CAD build for the part. Positions are in the model's coordinates, mm. Face numbers are marked on the shaded views. Give positions to 0.01 mm unless a question says otherwise; leave off trailing zeros. Loops run counter-clockwise (first coordinate to the right, second up) from the corner with the lowest first, then second, coordinate; pieces in that order, holes last.
Item 1: Mould opens along Z. For the marked faces 1, 2 and 3 say: released by +Z, released by -Z, zero draft, split by the parting line, or undercut.
Item 2: Saw through at C-C on x = -15.5. Give the cut face in (y, z).
Item 3: Saw through at B-B on z = 3. Give the cut face in (x, y), plus the area to 3 significant figures.
Item 4: Drop a flat-ended pin along its axis: P1, Ø4, axis at x = -15.5, z = -24.9, coming from the -Y side. Give the stop position or say it passes through.
Item 5: Probe probe 1 along X at (y, z) = (3.25, -14); probe 2 along Z at (x, y) = (25, 2.3); probe 3 along Z at (x, y) = (14.5, 4.5). List the from-to ranges inside material, lowest first.
Item 6: Saw through at A-A on x = -6.5. Give the cut face in (y, z).
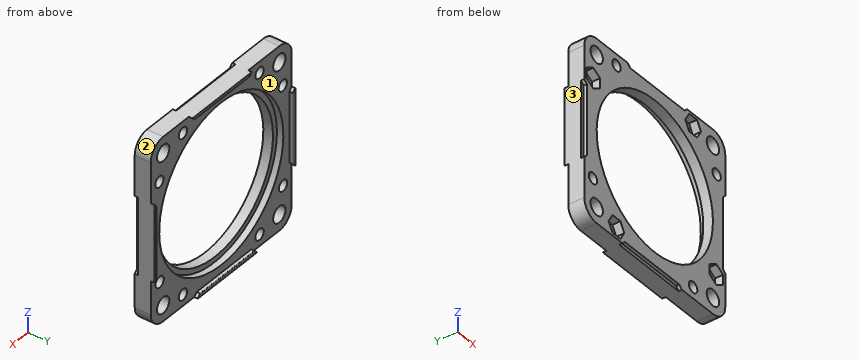
from build123d import *

# Parameters (mm, degrees)
BOSS_EXTRUDE1_DEPTH = 5
SKETCH2_R           = 1.7
SKETCH2_R_2         = 2.5
CUT_EXTRUDE3_DEPTH  = 5
SKETCH5_R           = 23.5
CUT_EXTRUDE5_DEPTH  = 41.614036982
SKETCH5_3_R         = 25.1
SKETCH5_3_R_2       = 23.5
CUT_EXTRUDE6_DEPTH  = 2
CUT_EXTRUDE7_START  = -2.5
SKETCH6_R           = 1.7
CUT_EXTRUDE7_DEPTH  = 2.5
BOSS_EXTRUDE2_DEPTH = 1.1
CUT_EXTRUDE8_DEPTH  = 1
CIRPATTERN9_COUNT   = 4
FILLET1_R           = 0.2


with BuildPart() as part:
    # Sketch1 → Boss-Extrude1 (new body)
    with BuildSketch(Plane(origin=(0, 0, 0), x_dir=(1, 0, 0), z_dir=(0, 1, 0))):
        with BuildLine():
            Line((23.5, -28.5), (-23.5, -28.5))
            ThreePointArc((-23.5, -28.5), (-27.035533906, -27.035533906), (-28.5, -23.5))
            Line((-28.5, -23.5), (-28.5, 23.5))
            ThreePointArc((-28.5, 23.5), (-27.035533906, 27.035533906), (-23.5, 28.5))
            Line((-23.5, 28.5), (23.5, 28.5))
            ThreePointArc((23.5, 28.5), (27.035533906, 27.035533906), (28.5, 23.5))
            Line((28.5, 23.5), (28.5, -23.5))
            ThreePointArc((28.5, -23.5), (27.035533906, -27.035533906), (23.5, -28.5))
        make_face()
    extrude(amount=BOSS_EXTRUDE1_DEPTH)

    # Sketch2 → Cut-Extrude3 (cut)
    with BuildSketch(Plane(origin=(0, 5, 0), x_dir=(1, 0, 0), z_dir=(0, 1, 0))):
        with Locations(Location((24.9, 15.5, 0), (0, 0, 270))):
            Circle(SKETCH2_R)
        with Locations(Location((15.5, 25, 0), (0, 0, 270))):
            Circle(SKETCH2_R)
        with Locations(Location((23.5, 23.5, 0), (0, 0, 270))):
            Circle(SKETCH2_R_2)
    cut_extrude3 = extrude(amount=-CUT_EXTRUDE3_DEPTH, mode=Mode.SUBTRACT)

    # Sketch5 → Cut-Extrude5 (cut, through all)
    with BuildSketch(Plane(origin=(0, 5, 0), x_dir=(1, 0, 0), z_dir=(0, 1, 0))):
        with Locations(Location((0, 0, 0), (0, 0, 270))):
            Circle(SKETCH5_R)
    extrude(amount=-CUT_EXTRUDE5_DEPTH, mode=Mode.SUBTRACT)

    # Sketch5<3> → Cut-Extrude6 (cut)
    with BuildSketch(Plane(origin=(0, 5, 0), x_dir=(1, 0, 0), z_dir=(0, 1, 0))):
        with Locations(Location((0, 0, 0), (0, 0, 270))):
            Circle(SKETCH5_3_R)
        with Locations(Location((0, 0, 0), (0, 0, 270))):
            Circle(SKETCH5_3_R_2, mode=Mode.SUBTRACT)
    extrude(amount=-CUT_EXTRUDE6_DEPTH, mode=Mode.SUBTRACT)

    # Sketch6 → Cut-Extrude7 (cut)
    with BuildSketch(Plane.XZ.offset(CUT_EXTRUDE7_START)):
        Polygon((22.15, -13.91228676), (22.15, -17.08771324), (24.9, -18.675426481), (27.65, -17.08771324), (27.65, -13.91228676), (24.9, -12.324573519), align=None)
        with Locations(Location((24.9, -15.5, 0), (0, 0, 90))):
            Circle(SKETCH6_R, mode=Mode.SUBTRACT)
    cut_extrude7 = extrude(amount=CUT_EXTRUDE7_DEPTH, mode=Mode.SUBTRACT)

    # Sketch7 → Boss-Extrude2 (add)
    with BuildSketch(Plane(origin=(0, 5, 0), x_dir=(1, 0, 0), z_dir=(0, 1, 0))):
        Polygon((-1.072782926, 27.5), (-1.072782926, 28.5), (-13.072782926, 28.5), (-12.072782926, 27.5), align=None)
        Polygon((9.927217074, 27.5), (10.927217074, 28.5), (-1.072782926, 28.5), (-1.072782926, 27.5), align=None)
    boss_extrude2 = extrude(amount=BOSS_EXTRUDE2_DEPTH)

    # Sketch8 → Cut-Extrude8 (cut)
    with BuildSketch(Plane.XZ):
        Polygon((-12.072782926, -27.5), (-13.072782926, -28.5), (10.927217074, -28.5), (9.927217074, -27.5), align=None)
    cut_extrude8 = extrude(amount=-CUT_EXTRUDE8_DEPTH, mode=Mode.SUBTRACT)

    # CirPattern9: Cut-Extrude3, Cut-Extrude7, Boss-Extrude2, Cut-Extrude8 ×4 about axis
    cirpattern9_axis = Axis((0, 0, 0), (0, 1, 0))
    add([cut_extrude3.rotate(cirpattern9_axis, i * 360 / CIRPATTERN9_COUNT) for i in range(1, CIRPATTERN9_COUNT)], mode=Mode.SUBTRACT)
    add([cut_extrude7.rotate(cirpattern9_axis, i * 360 / CIRPATTERN9_COUNT) for i in range(1, CIRPATTERN9_COUNT)], mode=Mode.SUBTRACT)
    add([boss_extrude2.rotate(cirpattern9_axis, i * 360 / CIRPATTERN9_COUNT) for i in range(1, CIRPATTERN9_COUNT)])
    add([cut_extrude8.rotate(cirpattern9_axis, i * 360 / CIRPATTERN9_COUNT) for i in range(1, CIRPATTERN9_COUNT)], mode=Mode.SUBTRACT)

    # Fillet1
    fillet1_edges = [part.edges().sort_by_distance(p)[0] for p in [
        (-27.5, 6.1, 1.072782926),
        (1.072782926, 6.1, 27.5),
        (27.5, 6.1, -1.072782926),
        (-1.072782926, 6.1, -27.5),
    ]]
    fillet(fillet1_edges, radius=FILLET1_R)


solid = part.part
Results below:
1. face 1: undercut
1. face 2: released by +Z
1. face 3: zero draft
2. outline: (0, -28.5) - (5, -28.5) - (5, -26.6) - (2.5, -26.6) - (2.5, -27.65) - (0, -27.65) - close; (0, -22.15) - (2.5, -22.15) - (2.5, -23.2) - (5, -23.2) - (5, -19.74) - (3, -19.74) - (3, -17.66) - (0, -17.66) - close; (0, 17.66) - (3, 17.66) - (3, 19.74) - (5, 19.74) - (5, 23.3) - (0, 23.3) - close; (0, 26.7) - (5, 26.7) - (5, 28.5) - (0, 28.5) - close
3. outline: (-28.5, 1) - (-27.5, 1) - (-27.5, 0) - (-23.31, 0) - (-23.31, 3) - (-24.92, 3) - (-24.92, 5) - (-27.5, 5) - (-27.5, 5.9) arc R0.2 ccw to (-27.7, 6.1) - (-28.5, 6.1) - close; (23.31, 0) - (27.5, 0) - (27.5, 1) - (28.5, 1) - (28.5, 6.1) - (27.7, 6.1) arc R0.2 ccw to (27.5, 5.9) - (27.5, 5) - (24.92, 5) - (24.92, 3) - (23.31, 3) - close
3. area: 45.7 mm2
4. P1: stops at y = 2.5
5. probe 1: x = -28.5 to -25.8, -24.2 to -20.83, 20.83 to 24.1, 25.7 to 28.5
5. probe 2: z = -28.27 to -25.5, -21.5 to -18.62, -12.38 to 13.8, 17.2 to 21.5, 25.5 to 28.27
5. probe 3: z = -28.5 to -26.37, -23.63 to -20.49, 20.49 to 23.53, 26.27 to 28.5
6. outline: (0, -27.5) - (1, -27.5) - (1, -28.5) - (6.1, -28.5) - (6.1, -27.7) arc R0.2 ccw to (5.9, -27.5) - (5, -27.5) - (5, -24.24) - (3, -24.24) - (3, -22.58) - (0, -22.58) - close; (0, 22.58) - (3, 22.58) - (3, 24.24) - (5, 24.24) - (5, 27.5) - (5.9, 27.5) arc R0.2 ccw to (6.1, 27.7) - (6.1, 28.5) - (1, 28.5) - (1, 27.5) - (0, 27.5) - close
